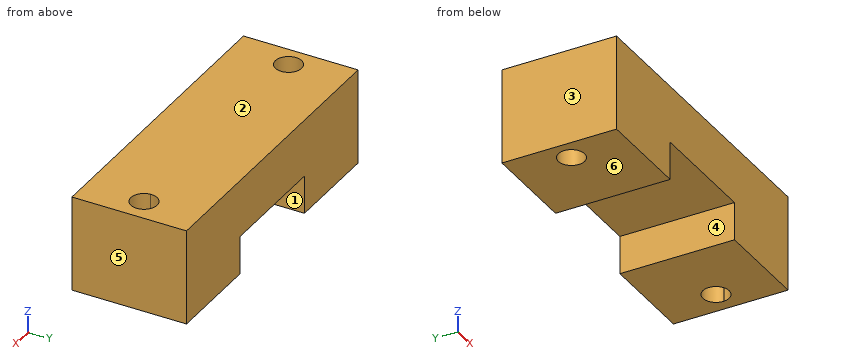
```python
from build123d import *

# Parameters (mm, degrees)
F0_W     = 80
F0_H     = 30
F1_DEPTH = 25
F2_W     = 30
F2_H     = 10
F3_DEPTH = 100
F5_DEPTH = 100
F6_R     = 3.439
F7_DEPTH = 100


with BuildPart() as f1:
    # F0 (on Top) → F1 (new body)
    with BuildSketch(Plane.XY):
        with Locations((-28.100313, 9.002365)):
            Rectangle(F0_W, F0_H)
    extrude(amount=F1_DEPTH)

    # F2 (on face) → F3 (cut)
    with BuildSketch(Plane.XZ.offset(5.997635)):
        with Locations((-28.100313, -5)):
            Rectangle(F2_W, F2_H)
        with Locations((-28.100313, 5)):
            Rectangle(F2_W, F2_H)
    extrude(amount=-F3_DEPTH, mode=Mode.SUBTRACT)

    # F4 (on face) → F5 (cut)
    with BuildSketch(Plane.XY.offset(25)):
        with BuildLine():
            ThreePointArc((8.935186, 9.280235), (5.357178, 12.716382), (2.068512, 9.002365))
            Line((2.068512, 9.002365), (8.923941, 9.002365))
            ThreePointArc((8.923941, 9.002365), (8.932373, 9.141186), (8.935186, 9.280235))
        make_face()
        with BuildLine():
            Line((8.923941, 9.002365), (2.068512, 9.002365))
            ThreePointArc((2.068512, 9.002365), (5.496227, 5.841276), (8.923941, 9.002365))
        make_face()
    extrude(amount=-F5_DEPTH, mode=Mode.SUBTRACT)

    # F6 (on face) → F7 (cut)
    with BuildSketch(Plane.XY.offset(25)):
        with Locations((-62.385514, 9.002365)):
            Circle(F6_R)
    extrude(amount=-F7_DEPTH, mode=Mode.SUBTRACT)


solid = f1.part
```
Geometry: final body of the model. Coordinates: model frame, mm. Face numbers are marked on the shaded views. A direction names the side the tool comes from. Round coordinates to 2 decimals unless told otherwise and drop trailing zeros. Write each loop counter-clockwise with the first axis right and the second up, starting at its lowest first coordinate (ties: lowest second). Pieces come first, ordered by that corner, then holes. Notation, with made-up numbers: M -6,52 L 17,52 A19 cw 17,57 Z; hole C 76.25,-19.5 d7. An arc over 180 degrees is marked long. Answer in a Markdown table with one row per item. Add a question column.
(1) Ray query, L1, parallel to X at y = -3.25, z = 4.75; L2, parallel to Z at x = -24, y = 20.5; L3, parallel to Y at x = 3, z = 19.5. Return the intervals inside material, ascending.
(2) Draft query along X for the marked faces 3, 4, 5 and 6. Return one class per face: pulls with the +X half, pulls with the -X half, needs draft (parallel to the pull), parting line crosses it, or undercut.
(3) Contact query for a flat-ended pin moving along its axis: pin 1 (6 mm diameter, centred on x = -28.5, y = 17.5, fed in from -Z). Output: stop coordinate, or through.
(4) Cut plane C-C, the plane x = 4. Return the cut outline in (y, z), then the cut area to 3 significant figures.
(5) Reachability of the marked faces 1 and 2 from +Z, -Z, +X, -X, +Y, -Y: full face, straight path, thin tool, end or side. Return the list, or none.
(6) Cut plane B-B, the plane y = 2.75. Return the cut outline in (x, z).
(7) Cut plane D-D, the plane z = 18.25. Return the cut outline in (x, y).
(8) Cut plane A-A, the plane z = 5.5. Return the cut outline in (x, y).
Established:
| question | item | result |
|---|---|---|
| 1 | L1 | -68.1 to -43.1, -13.1 to 11.9 |
| 1 | L2 | 10 to 25 |
| 1 | L3 | -6 to 6.91, 11.65 to 24 |
| 2 | face 3 | pulls with the -X half |
| 2 | face 4 | undercut |
| 2 | face 5 | pulls with the +X half |
| 2 | face 6 | needs draft |
| 3 | pin 1 | z = 10 |
| 4 | outline | M -6,0 L 6.18,0 L 6.18,25 L -6,25 Z; M 12.38,0 L 24,0 L 24,25 L 12.38,25 Z |
| 4 | area | 595 mm² |
| 5 | face 1 | -Z, +Y, -Y |
| 5 | face 2 | +Z, +X, -X, +Y, -Y |
| 6 | outline | M -68.1,0 L -43.1,0 L -43.1,10 L -13.1,10 L -13.1,0 L 11.9,0 L 11.9,25 L -68.1,25 Z |
| 7 | outline | M -68.1,-6 L 11.9,-6 L 11.9,24 L -68.1,24 Z; hole C -62.39,9 d6.88; hole M 8.92,9 A3.44 ccw 8.94,9.28 A3.44 ccw long Z |
| 8 | outline | M -68.1,-6 L -43.1,-6 L -43.1,24 L -68.1,24 Z; M -13.1,-6 L 11.9,-6 L 11.9,24 L -13.1,24 Z; hole C -62.39,9 d6.88; hole M 8.92,9 A3.44 ccw 8.94,9.28 A3.44 ccw long Z |
